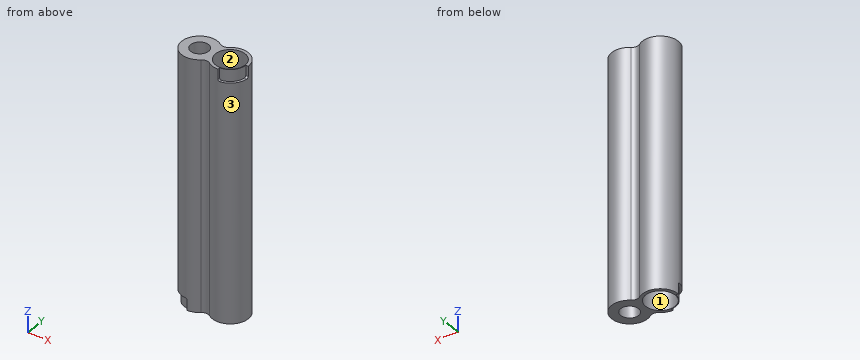
from build123d import *

# Parameters (mm, degrees)
BOSS_EXTRUDE1_DEPTH = 34.5
SKETCH2_R           = 4.125
CUT_EXTRUDE1_DEPTH  = 34.5
SKETCH3_R           = 4.125
SKETCH3_R_2         = 2.5
BOSS_EXTRUDE2_DEPTH = 3.25
SKETCH5_R           = 4.125
SKETCH5_R_2         = 2.5
BOSS_EXTRUDE4_DEPTH = 3.25
CUT_EXTRUDE3_DEPTH  = 3.25
FILLET1_R           = 0.5
CUT_EXTRUDE4_DEPTH  = 3.25
FILLET2_R           = 0.5


with BuildPart() as part:
    # Sketch1 → Boss-Extrude1 (new body, symmetric)
    with BuildSketch(Plane.XY):
        with BuildLine():
            ThreePointArc((2.986131566, 4.010363858), (-4.999610571, -0.062403009), (3.085297006, -3.934582873))
            ThreePointArc((3.085297006, -3.934582873), (4.294454604, -3.508571794), (5.513868434, -3.904270479))
            ThreePointArc((5.513868434, -3.904270479), (13.499610571, 0.168496387), (5.414702994, 4.040676252))
            ThreePointArc((5.414702994, 4.040676252), (4.205545396, 3.614665172), (2.986131566, 4.010363858))
        make_face()
    extrude(amount=BOSS_EXTRUDE1_DEPTH, both=True)

    # Sketch2 → Cut-Extrude1 (cut, symmetric)
    with BuildSketch(Plane.XY):
        Circle(SKETCH2_R)
        with Locations((8.5, 0.106093378)):
            Circle(SKETCH2_R)
    extrude(amount=CUT_EXTRUDE1_DEPTH, both=True, mode=Mode.SUBTRACT)

    # Sketch3 → Boss-Extrude2 (add)
    with BuildSketch(Plane.XY.offset(34.5)):
        Circle(SKETCH3_R)
        Circle(SKETCH3_R_2, mode=Mode.SUBTRACT)
    extrude(amount=-BOSS_EXTRUDE2_DEPTH)

    # Sketch5 → Boss-Extrude4 (add)
    with BuildSketch(Plane(origin=(0, 0, -34.5), x_dir=(-1, 0, 0), z_dir=(0, 0, -1))):
        with Locations((-8.5, 0.106093378)):
            Circle(SKETCH5_R)
        with Locations((-8.5, 0.106093378)):
            Circle(SKETCH5_R_2, mode=Mode.SUBTRACT)
    extrude(amount=-BOSS_EXTRUDE4_DEPTH)

    # Sketch6 → Cut-Extrude3 (cut)
    with BuildSketch(Plane(origin=(0, 0, -34.5), x_dir=(-1, 0, 0), z_dir=(0, 0, -1))):
        with BuildLine():
            Line((4.299610571, -0.062403009), (4.999610571, -0.062403009))
            ThreePointArc((4.999610571, -0.062403009), (3.513401838, -3.557528288), (0, -5))
            Line((0, -5), (0, -4.300063395))
            ThreePointArc((0, -4.300063395), (3.01846056, -3.062587313), (4.299610571, -0.062403009))
        make_face()
    extrude(amount=-CUT_EXTRUDE3_DEPTH, mode=Mode.SUBTRACT)

    # Fillet1
    fillet1_edges = [part.edges().sort_by_distance(p)[0] for p in [
        (0, -4.650031697, -31.25),
        (-4.649610571, -0.062403009, -31.25),
    ]]
    fillet(fillet1_edges, radius=FILLET1_R)

    # Sketch7 → Cut-Extrude4 (cut)
    with BuildSketch(Plane.XY.offset(34.5)):
        with BuildLine():
            Line((13.5, 0.106093378), (12.8, 0.106093378))
            ThreePointArc((12.8, 0.106093378), (11.540559159, -2.934465781), (8.5, -4.193906622))
            Line((8.5, -4.193906622), (8.5, -4.893906622))
            ThreePointArc((8.5, -4.893906622), (12.035533906, -3.429440528), (13.5, 0.106093378))
        make_face()
    extrude(amount=-CUT_EXTRUDE4_DEPTH, mode=Mode.SUBTRACT)

    # Fillet2
    fillet2_edges = [part.edges().sort_by_distance(p)[0] for p in [
        (8.5, -4.543906622, 31.25),
        (13.15, 0.106093378, 31.25),
    ]]
    fillet(fillet2_edges, radius=FILLET2_R)


solid = part.part
For this review, take the finished solid that the model builds, in its own axes (mm). Face numbers are marked on the shaded views. A direction names the side the tool comes from. Round coordinates to 2 decimals unless told otherwise and drop trailing zeros. Order: outer loops, then holes, each group sorted by start corner. A loop starts at its lowest first (then second) coordinate and runs counter-clockwise, first axis right, second up. Notation, with made-up numbers: (38, -0.75) -> (89, -0.75) arc R15 cw to (89, 17.25) -> close; hole circle Ø3 at (12.5, 59.5). An arc over 180 degrees is marked (long way). Write item = value, one per line. Start each with the question number.
1) Tool access review of the marked faces 1, 2 and 3: name each direction out of +Z, -Z, +X, -X, +Y, -Y from which nothing blocks a thin tool from reaching the whole face with its end or side.
2) Take a section at A-A on x = 1.75. State the section outline as (y, z) points, plus the area to 3 significant figures.
3) To check wall thickness, follow line 1 (Y direction, x = 0, z = 32); line 2 (Y direction, x = 0, z = 0.5) (3 decimals); line 3 (X direction, y = 0.75, z = -5). State the ranges of each line that lie inside material, in increasing order. Write a range as from..to.
4) Take a section at B-B on z = -15. Count the separate pieces of the cut face and the enclosed holes in it, plus the area to 3 significant figures.
5) Insertion check: pin 1 (4.5 mm diameter, centred on x = 8.5, y = 0.11, fed in from -Z); pin 2 (4 mm diameter, centred on y = -0.5, z = 13.5, fed in from -X); pin 3 (1 mm diameter, centred on y = 2, z = 3, fed in from +X). Each pin has a flat end and moves straight along its axis. Give the tip position at first contact, or say it passes through.
6) Take a section at C-C on x = -3.5. State the section outline as (y, z) points, plus the area to 3 significant figures.
Verdict:
q1.face_1 = -Z
q1.face_2 = +Z
q1.face_3 = +Z, -Z
q2.outline = (-4.68, -34.5) -> (-3.74, -34.5) -> (-3.74, 31.25) -> (-1.79, 31.25) -> (-1.79, 34.5) -> (-4.68, 34.5) -> close; (1.79, 31.25) -> (3.74, 31.25) -> (3.74, -34.5) -> (4.68, -34.5) -> (4.68, 34.5) -> (1.79, 34.5) -> close
q2.area = 144 mm2
q3.line_1 = -5..-2.5, 2.5..5
q3.line_2 = -5..-4.125, 4.125..5
q3.line_3 = -4.94..-4.06, 4.06..4.43, 12.57..13.46
q4.separate_pieces = 1
q4.enclosed_holes = 2
q4.area = 46.3 mm2
q5.pin_1 = through
q5.pin_2 = -5
q5.pin_3 = 13.3
q6.outline = (-3.57, -31.25) -> (-2.5, -31.25) -> (-2.5, -34.5) -> (-2.18, -34.5) -> (-2.18, 31.25) -> (2.18, 31.25) -> (2.18, -34.5) -> (3.57, -34.5) -> (3.57, 34.5) -> (-3.57, 34.5) -> close
q6.area = 202 mm2
